```python
from build123d import *

# Parameters (mm, degrees)
F0_R     = 42.2402
F1_DEPTH = 96.901
F2_R     = 3.9497
F3_DEPTH = 30.48
F4_R     = 2.0955
F5_DEPTH = 11.938
F7_DEPTH = 16.51


with BuildPart() as f1:
    # F0 (on Front) → F1 (new body)
    with BuildSketch(Plane.XZ):
        Circle(F0_R)
    extrude(amount=F1_DEPTH)

    # F2 (on face) → F3 (join)
    with BuildSketch(Plane.XZ.offset(96.901)):
        Circle(F2_R)
    extrude(amount=F3_DEPTH)

    # F4 (on face) → F5 (join)
    with BuildSketch(Plane.XZ.offset(96.901)):
        with Locations((-36.195, 0)):
            Circle(F4_R)
        with Locations((36.195, 0)):
            Circle(F4_R)
    extrude(amount=F5_DEPTH)

    # F6 (on face) → F7 (cut)
    with BuildSketch(Plane.XZ.offset(127.381)):
        with BuildLine():
            Line((-2.7789503774, -2.8067), (-4.5821680687, -2.8067))
            Line((-4.5821680687, -2.8067), (-4.5821680687, -6.1287720943))
            Line((-4.5821680687, -6.1287720943), (4.5821680687, -6.1287720943))
            Line((4.5821680687, -6.1287720943), (4.5821680687, -2.8067))
            Line((4.5821680687, -2.8067), (2.7789503774, -2.8067))
            ThreePointArc((2.7789503774, -2.8067), (0, -3.9497), (-2.7789503774, -2.8067))
        make_face()
        with BuildLine():
            Line((2.7789503774, -2.8067), (-2.7789503774, -2.8067))
            ThreePointArc((-2.7789503774, -2.8067), (0, -3.9497), (2.7789503774, -2.8067))
        make_face()
    extrude(amount=-F7_DEPTH, mode=Mode.SUBTRACT)


solid = f1.part
```
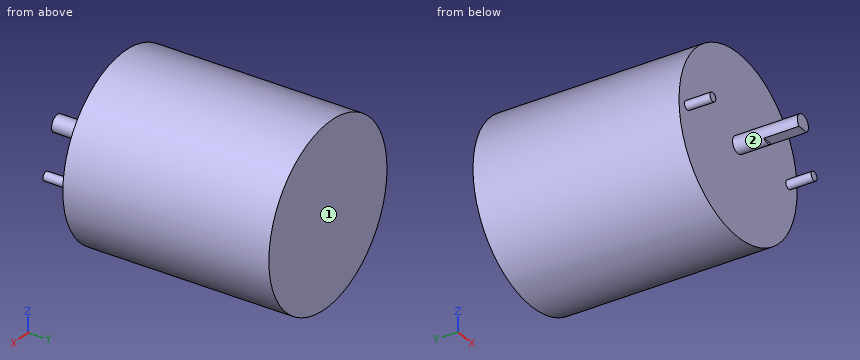
CAD build for the part. Positions are in the model's coordinates, mm. Face numbers are marked on the shaded views. A direction names the side the tool comes from. Round coordinates to 2 decimals unless told otherwise and drop trailing zeros. Order: outer loops, then holes, each group sorted by start corner. A loop starts at its lowest first (then second) coordinate and runs counter-clockwise, first axis right, second up.
Item 1: Pin check, flat tips, straight feed: pin 1 (8 mm diameter, centred on y = -67, z = 27, fed in from -X); pin 2 (5 mm diameter, centred on x = 22.5, y = -84.5, fed in from -Z); pin 3 (4.5 mm diameter, centred on x = 0, y = -116, fed in from -Z); pin 4 (3 mm diameter, centred on x = 25, z = 29, fed in from +Y). Stop position of each tip, or through.
Item 2: Saw through at A-A on z = 0. Write the cut outline in (x, y), then the cut area to 3 significant figures.
Item 3: Probe line 1 along Y through (x, z) = (-19, 11); line 2 along Z through (x, y) = (-0.5, -58); line 3 along X through (y, z) = (-73, 37). List the from-to ranges inside material, lowest first.
Item 4: Saw through at B-B on y = -107. Write the cut outline in (x, z) (1 decimal), then the cut area to 3 significant figures.
Item 5: Tool access for the marked faces 1 and 2: list every direction of +Z, -Z, +X, -X, +Y, -Y with a clear straight run to the whole face (end or side of a thin tool).
Item 6: Saw through at D-D on y = -83. Write the cut outline in (x, z), then the cut area to 3 significant figures.
Item 7: Saw through at C-C on x = 0. Write the cut outline in (y, z), then the cut area to 3 significant figures.
Reported:
1. pin 1: stops at x = -35.43
1. pin 2: stops at z = -37.21
1. pin 3: stops at z = -2.81
1. pin 4: stops at y = 0
2. outline: (-42.24, -96.9) - (-38.29, -96.9) - (-38.29, -108.84) - (-34.1, -108.84) - (-34.1, -96.9) - (-3.95, -96.9) - (-3.95, -127.38) - (3.95, -127.38) - (3.95, -96.9) - (34.1, -96.9) - (34.1, -108.84) - (38.29, -108.84) - (38.29, -96.9) - (42.24, -96.9) - (42.24, 0) - (-42.24, 0) - close
2. area: 8,530 mm2
3. line 1: y = -96.9 to 0
3. line 2: z = -42.24 to 42.24
3. line 3: x = -20.38 to 20.38
4. outline: circle Ø4.2 at (-36.2, 0); circle Ø7.9 at (0, 0); circle Ø4.2 at (36.2, 0)
4. area: 76.6 mm2
5. face 1: +Z, -Z, +X, -X, +Y
5. face 2: -Y
6. outline: circle Ø84.48 at (0, 0)
6. area: 5,610 mm2
7. outline: (-127.38, -2.81) - (-110.87, -2.81) - (-110.87, -3.95) - (-96.9, -3.95) - (-96.9, -42.24) - (0, -42.24) - (0, 42.24) - (-96.9, 42.24) - (-96.9, 3.95) - (-127.38, 3.95) - close
7. area: 8,410 mm2
